Verification items for the finished model (mm, model axes). A direction names the side the tool comes from. Give positions to 0.01 mm unless a question says otherwise; leave off trailing zeros. Write each loop counter-clockwise with the first axis right and the second up, starting at its lowest first coordinate (ties: lowest second). Pieces come first, ordered by that corner, then holes.
from build123d import *

# Parameters (mm, degrees)
F0_R     = 6.35
F1_DEPTH = 7.62


with BuildPart() as f1:
    # F0 (on Front) → F1 (new body)
    with BuildSketch(Plane.XZ):
        Circle(F0_R)
        with BuildLine():
            ThreePointArc((4.408108, 0.5715), (4.435767, 0.286345), (4.445, 0))
            ThreePointArc((4.445, 0), (4.435767, -0.286345), (4.408108, -0.5715))
            ThreePointArc((4.408108, -0.5715), (3.14309, -3.14309), (0.5715, -4.408108))
            ThreePointArc((0.5715, -4.408108), (0, -4.445), (-0.5715, -4.408108))
            ThreePointArc((-0.5715, -4.408108), (-3.14309, -3.14309), (-4.408108, -0.5715))
            ThreePointArc((-4.408108, -0.5715), (-4.445, 0), (-4.408108, 0.5715))
            ThreePointArc((-4.408108, 0.5715), (-3.14309, 3.14309), (-0.5715, 4.408108))
            ThreePointArc((-0.5715, 4.408108), (0, 4.445), (0.5715, 4.408108))
            ThreePointArc((0.5715, 4.408108), (3.14309, 3.14309), (4.408108, 0.5715))
        make_face(mode=Mode.SUBTRACT)
        with BuildLine():
            Line((0.5715, 3.823908), (0.5715, 4.408108))
            ThreePointArc((0.5715, 4.408108), (0, 4.445), (-0.5715, 4.408108))
            Line((-0.5715, 4.408108), (-0.5715, 3.823908))
            Line((-0.5715, 3.823908), (0.5715, 3.823908))
        make_face()
        with BuildLine():
            ThreePointArc((4.408108, -0.5715), (4.435767, -0.286345), (4.445, 0))
            ThreePointArc((4.445, 0), (4.435767, 0.286345), (4.408108, 0.5715))
            Line((4.408108, 0.5715), (3.823908, 0.5715))
            Line((3.823908, 0.5715), (3.823908, -0.5715))
            Line((3.823908, -0.5715), (4.408108, -0.5715))
        make_face()
        with BuildLine():
            ThreePointArc((-0.5715, -4.408108), (0, -4.445), (0.5715, -4.408108))
            Line((0.5715, -4.408108), (0.5715, -3.823908))
            Line((0.5715, -3.823908), (-0.5715, -3.823908))
            Line((-0.5715, -3.823908), (-0.5715, -4.408108))
        make_face()
        with BuildLine():
            Line((-3.823908, 0.5715), (-4.408108, 0.5715))
            ThreePointArc((-4.408108, 0.5715), (-4.445, 0), (-4.408108, -0.5715))
            Line((-4.408108, -0.5715), (-3.823908, -0.5715))
            Line((-3.823908, -0.5715), (-3.823908, 0.5715))
        make_face()
    extrude(amount=F1_DEPTH)


solid = f1.part
Item 1: Scan lines: line 1 along Z through (x, y) = (4, -1.75); line 2 along Z through (x, y) = (2.25, -1); line 3 along X through (y, z) = (-6.5, -3). Record each from-to range of solid material in increasing order.
Answer key:
line 1: z = -4.93 to -1.94, -0.57 to 0.57, 1.94 to 4.93
line 2: z = -5.94 to -3.83, 3.83 to 5.94
line 3: x = -5.6 to -3.28, 3.28 to 5.6
Item 2: Release check for a two-part mould opening along X. For faces 3 (the face through (0, -7.62, -4)), 4 (the face through (0, -4, -3.824)), 5 (the face through (-1.38, -3.76, -6.2)) record: released by +X, released by -X, zero draft, split by the parting line, or undercut.
Answer key:
face 3: zero draft
face 4: undercut
face 5: split by the parting line
Item 3: Sectioned sample at B-B on z = 0. Record the cut outline in (x, y), then the cut area to 3 significant figures.
Answer key:
outline: (-6.35, -7.62) - (-3.82, -7.62) - (-3.82, 0) - (-6.35, 0) - close; (3.82, -7.62) - (6.35, -7.62) - (6.35, 0) - (3.82, 0) - close
area: 38.5 mm2
Item 4: Set-up check for faces 1 (the face through (3.172, -3.757, -3.114)), 2 (the face through (0, 0, -4)): record each of +Z, -Z, +X, -X, +Y, -Y from which the full face is reachable in a straight line by a thin tool's end or side.
Answer key:
face 1: +Y, -Y
face 2: +Z, -Z, +X, -X, +Y
Item 5: Sectioned sample at C-C on x = 0. Record the cut outline in (y, z), then the cut area to 3 significant figures.
Answer key:
outline: (-7.62, -6.35) - (0, -6.35) - (0, -3.82) - (-7.62, -3.82) - close; (-7.62, 3.82) - (0, 3.82) - (0, 6.35) - (-7.62, 6.35) - close
area: 38.5 mm2
Item 6: Depth check by flat-ended pin: pin 1 (0.5 mm diameter, centred on x = 4, y = -3, fed in from +Z); pin 2 (3 mm diameter, centred on x = -4.5, y = -6.5, fed in from +Z); pin 3 (0.6 mm diameter, centred on x = -4, y = -5.5, fed in from +Z). Enter the tip coordinate at first touch or a pass-through.
Answer key:
pin 1: stops at z = 5.12
pin 2: stops at z = 5.6
pin 3: stops at z = 5.16
Item 7: Sectioned sample at D-D on x = 5.25. Record the cut outline in (y, z), then the cut area to 3 significant figures.
Answer key:
outline: (-7.62, -3.57) - (0, -3.57) - (0, 3.57) - (-7.62, 3.57) - close
area: 54.4 mm2
